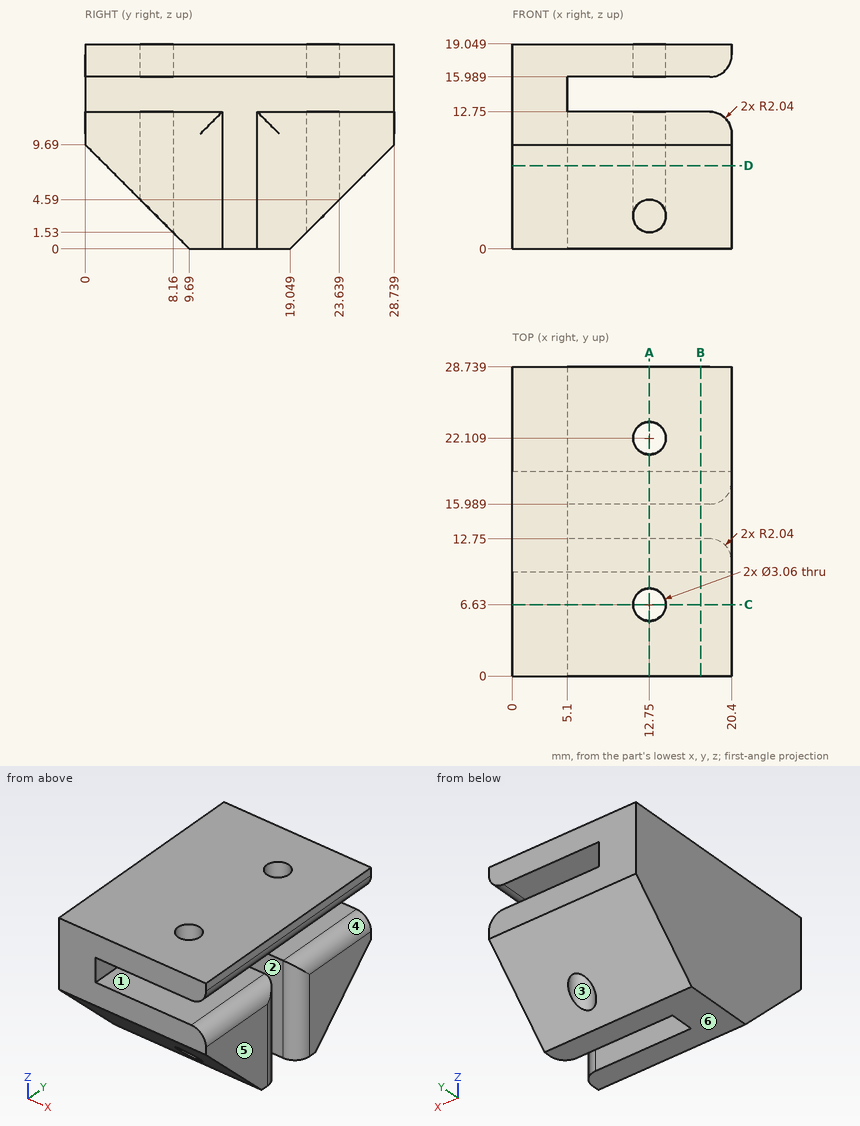
The drawing under review shows one solid part. Ordinate dimensions are in mm from its lowest x, y, z. A direction names the side the tool comes from. Coordinates: 2 decimals unless noted, no trailing zeros. Order: outer loops, then holes, each group sorted by start corner. A loop starts at its lowest first (then second) coordinate and runs counter-clockwise, first axis right, second up. Notation, with made-up numbers: M -3.75,20.5 L 32.25,20.5 A9 ccw 32.25,28.5 Z; hole C 81.5,34 d7. An arc over 180 degrees is marked long. One line per question, with ' | ' between items.
(1) Add section A-A, the plane x = 12.75. State how many separate pieces and enclosed holes the cut face has, then the cut area to 3 significant figures.
Geometry results:
separate pieces: 7 | enclosed holes: 0 | area: 241 mm²
(2) Add section D-D, the plane z = 7.75. Write out the cut boundary in (x, y), then the cut area to 3 significant figures.
Geometry results:
outline: M 0,1.94 L 20.4,1.94 L 20.4,10.71 A2.04 ccw 18.36,12.75 L 5.1,12.75 L 5.1,15.99 L 18.36,15.99 A2.04 ccw 20.4,18.03 L 20.4,26.8 L 0,26.8 Z; hole C 12.75,6.63 d3.06; hole C 12.75,22.11 d3.06 | area: 441 mm²
(3) Insertion check: pin 1 (1.8 mm diameter, centred on x = 12.75, y = 22.11, fed in from -Z); pin 2 (10 mm diameter, centred on x = 16, z = 13, fed in from -Y); pin 3 (6.5 mm diameter, centred on x = 10, z = 5.5, fed in from +Y); pin 4 (5 mm diameter, centred on x = 12.75, y = 22.11, fed in from -Z). Each pin has a flat end and moves straight along its axis. Give the tip position at first contact, or say it passes through.
Geometry results:
pin 1: passes through | pin 2: stops at y = 0 | pin 3: stops at y = 27.8 | pin 4: stops at z = 0.56
(4) Add section C-C, the plane y = 6.63. Write out the cut boundary in (x, z), then the cut area to 3 significant figures.
Geometry results:
outline: M 0,3.06 L 11.22,3.06 L 11.22,12.75 L 5.1,12.75 L 5.1,15.99 L 11.22,15.99 L 11.22,19.05 L 0,19.05 Z; M 14.28,3.06 L 20.4,3.06 L 20.4,10.71 A2.04 ccw 18.36,12.75 L 14.28,12.75 Z; M 14.28,15.99 L 18.36,15.99 A2.04 ccw 20.4,18.03 L 20.4,19.05 L 14.28,19.05 Z | area: 236 mm²
(5) Machinability: for the marked faces 1, 2 and 3, which of the approach directions +Z, -Z, +X, -X, +Y, -Y give a long, thin tool a straight path to every point of the face, cutting with its end or side? Answer none if there is none.
Geometry results:
face 1: +X, +Y, -Y | face 2: -Z, +X | face 3: +Z, -Z
(6) For probe 1 along Y at (x, z) = (12.75, 17.05); probe 2 along Y at (x, z) = (18.5, 10.5) (1 decimal); probe 3 along Z at (x, y) = (15.75, 19), list the stretches that pass through material, from the lowest coordinate up. Write a range as from..to.
Geometry results:
probe 1: y = 0..5.1, 8.16..20.58, 23.64..28.74 | probe 2: y = 0..12.7, 16..28.7 | probe 3: z = 0..12.75, 15.99..19.05
(7) The part is to be moulded in two halves that separate along Z. For the marked faces 4, 5 and 6, say which applies: +Z half, -Z half, draft (parallel to the pull), parting line (faces both ways), or undercut.
Geometry results:
face 4: undercut | face 5: draft | face 6: -Z half
(8) Add section B-B, the plane x = 17.5. Write out the cut boundary in (y, z).
Geometry results:
outline: M 0,9.69 L 9.69,0 L 12.75,0 L 12.75,12.75 L 0,12.75 Z; M 0,15.99 L 28.74,15.99 L 28.74,19.05 L 0,19.05 Z; M 15.99,0 L 19.05,0 L 28.74,9.69 L 28.74,12.75 L 15.99,12.75 Z
